Autodesk Inventor part; units mm, degrees
ref_plane "YZ Plane" through (0, 0, 0) normal (1, 0, 0) x (0, 1, 0)
ref_plane "XZ Plane" through (0, 0, 0) normal (0, 1, 0) x (-1, 0, 0)
ref_plane "XY Plane" through (0, 0, 0) normal (0, 0, 1) x (1, 0, 0)
ref_plane "Work Plane1" through (0, 0, 0) normal (0, 0, 1) x (1, 0, 0)
sketch "Sketch1" plane through (0, 0, 0) normal (0, 0, 1) x (1, 0, 0)
  line L0 (14.7416, 30.2896) -> (14.7416, 47.46)
  line L1 (14.7416, 29.7816) -> (14.7416, 30.2896)
  line L2 (14.7416, -47.4598) -> (14.7416, 29.7816)
  arc A0 (14.7416, 47.46) -> (12.2016, 50) centre (12.2016, 47.46) ccw
  line L3 (12.2016, 50) -> (-68.0116, 50)
  arc A1 (12.2016, -49.9998) -> (14.7416, -47.4598) centre (12.2016, -47.4598) ccw
  line L4 (-6.315, -49.9998) -> (12.2016, -49.9998)
  line L5 (-157.7498, -49.9998) -> (-92.5988, -49.9998)
  line L6 (-269.9924, -49.9998) -> (-263.9218, -49.9998)
  line L7 (-263.9218, -49.9998) -> (-241.9762, -49.9998)
  arc A2 (-280, -39.9922) -> (-269.9924, -49.9998) centre (-269.9924, -39.9922) ccw
  line L8 (-280, 39.2304) -> (-280, -39.9922)
  arc A3 (-269.9924, 50) -> (-280, 39.9924) centre (-269.9924, 39.9924) ccw
  line L9 (-280, 39.9924) -> (-280, 39.2304)
  line L10 (-263.4646, 50) -> (-269.9924, 50)
  line L11 (-152.238, 50) -> (-263.4646, 50)
  line L12 (-152.238, 50) -> (-68.0116, 50)
  line L13 (-92.5988, -49.9998) -> (-6.315, -49.9998)
  line L14 (-157.7498, -49.9998) -> (-241.9762, -49.9998)
  point P0 (0, 0)
extrude "Extrusion1" add sketch "Sketch1" along normal blind 1.6
sketch "Sketch2" plane through (0, 0, 1.6) normal (0, 0, 1) x (1, 0, 0)
  circle A0 centre (0.1366, 35.649) radius 1.75
  circle A1 centre (-13.046, 44.1326) radius 1.75
  circle A2 centre (0.1366, -38.011) radius 1.75
  circle A3 centre (-13.046, -44.107) radius 1.75
  circle A4 centre (-73.2948, 44.1072) radius 1.75
  circle A5 centre (-86.706, -44.107) radius 1.75
  circle A6 centre (-146.9548, 44.1072) radius 1.75
  circle A7 centre (-163.033, -44.107) radius 1.75
  circle A8 centre (-250.0026, -44.107) radius 1.75
  circle A9 centre (-271.3132, -38.011) radius 1.75
  circle A10 centre (-236.693, -44.107) radius 1.75
  circle A11 centre (-271.3132, 35.649) radius 1.75
  circle A12 centre (-250.0026, 44.1326) radius 1.75
  point P0 (0, 0)
hole "Hole1" at (0.1366, 35.649, 1.6) at (-13.046, 44.1326, 1.6) at (0.1366, -38.011, 1.6) at (-13.046, -44.107, 1.6) at (-86.706, -44.107, 1.6) at (-146.9548, 44.1072, 1.6) at (-163.033, -44.107, 1.6) at (-236.693, -44.107, 1.6) at (-250.0026, -44.107, 1.6) at (-271.3132, -38.011, 1.6) at (-271.3132, 35.649, 1.6) at (-250.0026, 44.1326, 1.6) at (-73.2948, 44.1072, 1.6) direction (0, 0, -1) diameter 1.6 depth 5 tip angle 118
sketch "Sketch3" plane through (0, 0, 1.6) normal (0, 0, 1) x (1, 0, 0)
  line L0 (8.922, 31.9915) -> (8.922, -34.5585)
  line L1 (-0.978, 31.9915) -> (8.922, 31.9915)
  line L2 (-0.978, 31.9915) -> (-0.978, -34.5585)
  line L3 (8.922, -34.5585) -> (-0.978, -34.5585)
  line L4 (-76.7473, 52.8925) -> (-76.7473, 42.9925)
  line L5 (-143.2973, 52.8925) -> (-76.7473, 52.8925)
  line L6 (-143.2973, 42.9925) -> (-76.7473, 42.9925)
  line L7 (-143.2973, 42.9925) -> (-143.2973, 52.8925)
  line L8 (-16.7036, -42.9923) -> (-16.7036, -52.8923)
  line L9 (-16.7036, -52.8923) -> (-83.2536, -52.8923)
  line L10 (-16.7036, -42.9923) -> (-83.2536, -42.9923)
  line L11 (-83.2536, -52.8923) -> (-83.2536, -42.9923)
  line L12 (-166.6905, -42.9923) -> (-233.2405, -42.9923)
  line L13 (-166.6905, -52.8923) -> (-233.2405, -52.8923)
  line L14 (-233.2405, -52.8923) -> (-233.2405, -42.9923)
  line L15 (-166.6905, -42.9923) -> (-166.6905, -52.8923)
  line L16 (-262.5279, 31.9915) -> (-262.5279, -34.5585)
  line L17 (-272.4279, 31.9915) -> (-262.5279, 31.9915)
  line L18 (-272.4279, 31.9915) -> (-272.4279, -34.5585)
  line L19 (-262.5279, -34.5585) -> (-272.4279, -34.5585)
  point P0 (0, 0)
extrude "Extrusion2" cut sketch "Sketch3" against normal blind 1.6
properties part number "Spacing Layer 4"
Could you check a few things on this model? Use its own coordinates, in mm. Coordinates: 2 decimals unless noted, no trailing zeros. Order: outer loops, then holes, each group sorted by start corner. A loop starts at its lowest first (then second) coordinate and runs counter-clockwise, first axis right, second up.
Q1. Suppose I cut it at B-B on x = -181. Please give me the cut outline in (y, z), and give its area (3 significant figures).
Q2. Will these pins go through, and if not, where does the flat tip stop? pin 1 (0.8 mm diameter, centred on y = -47.5, z = 0.5, fed in from -X); pin 2 (1.3 mm diameter, centred on x = 0.14, y = 35.65, fed in from +Z); pin 3 (0.5 mm diameter, centred on x = -64.5, z = 0.5, fed in from -Y); pin 4 (0.8 mm diameter, centred on y = 46, z = 0.5, fed in from -X).
Q3. Please list where these lines run through material, in increasing order: L1, parallel to X at y = 12, z = 0.35; L2, parallel to Y at x = -229, z = 0.55; L3, parallel to Y at x = -97.5, z = 0.85.
Q4. Suppose I cut it at C-C on z = 0.5. Give the number of separate pieces and of enclosed holes in the cut face, and give its area (3 significant figures).
Q5. Suppose I cut it at A-A on y = -5. Please give me the cut outline in (x, z).
Answer:
1. outline: (-42.99, 0) - (50, 0) - (50, 1.6) - (-42.99, 1.6) - close
1. area: 149 mm2
2. pin 1: stops at x = -277.04
2. pin 2: passes through
2. pin 3: stops at y = -42.99
2. pin 4: stops at x = -278.28
3. L1: x = -280 to -272.43, -262.53 to -0.98, 8.92 to 14.74
3. L2: y = -42.99 to 50
3. L3: y = -50 to 42.99
4. separate pieces: 1
4. enclosed holes: 15
4. area: 26,700 mm2
5. outline: (-280, 0) - (-272.43, 0) - (-272.43, 1.6) - (-280, 1.6) - close; (-262.53, 0) - (-0.98, 0) - (-0.98, 1.6) - (-262.53, 1.6) - close; (8.92, 0) - (14.74, 0) - (14.74, 1.6) - (8.92, 1.6) - close
